Source: CAD feature listing. Evaluate the final solid. Frame: model axes, mm. A direction names the side the tool comes from. Give positions to 0.01 mm unless a question says otherwise; leave off trailing zeros. Loops run counter-clockwise (first coordinate to the right, second up) from the corner with the lowest first, then second, coordinate; pieces in that order, holes last.
from build123d import *

# Parameters (mm, degrees)
ESQUISSE1_W             = 25
ESQUISSE1_H             = 20
ESQUISSE1_R             = 1.4
ESQUISSE1_R_2           = 0.875
BOSS_EXTRU_1_DEPTH      = 3
BOSS_EXTRU_2_DEPTH      = 6
ENL_V_MAT_EXTRU_1_DEPTH = 6
ESQUISSE4_R             = 2
ENL_V_MAT_EXTRU_2_DEPTH = 1
CONG_1_R                = 0.5
ESQUISSE5_R             = 1.4
ENL_V_MAT_EXTRU_3_DEPTH = 6


with BuildPart() as part:
    # Esquisse1 → Boss.-Extru.1 (new body)
    with BuildSketch(Plane.XY):
        with Locations((12.5, 10)):
            Rectangle(ESQUISSE1_W, ESQUISSE1_H)
        with Locations((22.5, 17.5)):
            Circle(ESQUISSE1_R, mode=Mode.SUBTRACT)
        with Locations((14.491447915, 8)):
            Circle(ESQUISSE1_R_2, mode=Mode.SUBTRACT)
        with Locations((7.991447915, 8)):
            Circle(ESQUISSE1_R_2, mode=Mode.SUBTRACT)
    extrude(amount=BOSS_EXTRU_1_DEPTH)

    # Esquisse2 → Boss.-Extru.2 (add)
    with BuildSketch(Plane.XY.offset(3)):
        with BuildLine():
            Line((0, 2), (1.8, 2))
            Line((1.8, 2), (1.8, 12.222275421))
            ThreePointArc((1.8, 12.222275421), (2.092893219, 12.929382202), (2.8, 13.222275421))
            Line((2.8, 13.222275421), (4.491447915, 13.222275421))
            Line((4.491447915, 13.222275421), (4.491447915, 2.730724668))
            Line((4.491447915, 2.730724668), (17.991447915, 2.730724668))
            Line((17.991447915, 2.730724668), (17.991447915, 12.493838982))
            Line((17.991447915, 12.493838982), (25, 12.493838982))
            Line((25, 12.493838982), (25, 0))
            Line((25, 0), (0, 0))
            Line((0, 0), (0, 2))
        make_face()
    extrude(amount=BOSS_EXTRU_2_DEPTH)

    # Esquisse3 → Enlèv. mat.-Extru.1 (cut)
    with BuildSketch(Plane(origin=(0, 2.730724668, 0), x_dir=(1, 0, 0), z_dir=(0, 1, 0))):
        with BuildLine():
            Line((9.692490841, -8.5), (9.692490841, -7))
            ThreePointArc((9.692490841, -7), (9.838937451, -6.646446609), (10.192490841, -6.5))
            Line((10.192490841, -6.5), (10.692490841, -6.5))
            ThreePointArc((10.692490841, -6.5), (11.046044232, -6.646446609), (11.192490841, -7))
            Line((11.192490841, -7), (11.192490841, -8.5))
            ThreePointArc((11.192490841, -8.5), (11.046044232, -8.853553391), (10.692490841, -9))
            Line((10.692490841, -9), (10.192490841, -9))
            ThreePointArc((10.192490841, -9), (9.838937451, -8.853553391), (9.692490841, -8.5))
        make_face()
    extrude(amount=-ENL_V_MAT_EXTRU_1_DEPTH, mode=Mode.SUBTRACT)

    # Esquisse4 → Enlèv. mat.-Extru.2 (cut)
    with BuildSketch(Plane.ZY.offset(-1.8)):
        with Locations((6, 8)):
            Circle(ESQUISSE4_R)
    extrude(amount=-ENL_V_MAT_EXTRU_2_DEPTH, mode=Mode.SUBTRACT)

    # Congé1
    cong_1_edges = [part.edges().sort_by_distance(p)[0] for p in [
        (12.5, 20, 0),
        (25, 10, 0),
        (12.5, 0, 0),
        (0, 10, 0),
        (0, 20, 1.5),
        (25, 20, 1.5),
        (25, 0, 4.5),
        (0, 0, 4.5),
    ]]
    fillet(cong_1_edges, radius=CONG_1_R)

    # Esquisse5 → Enlèv. mat.-Extru.3 (cut)
    with BuildSketch(Plane.XZ):
        with Locations(Location((21.12309895, 5.598466424, 0), (0, 0, 270))):
            Circle(ESQUISSE5_R)
    extrude(amount=-ENL_V_MAT_EXTRU_3_DEPTH, mode=Mode.SUBTRACT)


solid = part.part
1) Reachability of faces 1 (the flat face through (1.8, 6, 5)), 2 (the flat face through (21, 6, 6)), 3 (the flat face through (9.692, 1, 8)), 4 (the flat face through (12, 11, 3)) from +Z, -Z, +X, -X, +Y, -Y: full face, straight path, thin tool, end or side. Return the list, or none.
Checks:
face 1: +Z, -X, +Y
face 2: -Y
face 3: +Y, -Y
face 4: +Z, +Y
2) Cut plane D-D (z = 4.5). Return loops of the section in (x, y).
Checks:
outline: (0, 0.5) arc R0.5 ccw to (0.5, 0) - (20.26, 0) - (20.26, 6) - (21.99, 6) - (21.99, 0) - (24.5, 0) arc R0.5 ccw to (25, 0.5) - (25, 12.49) - (17.99, 12.49) - (17.99, 2.73) - (4.49, 2.73) - (4.49, 13.22) - (2.8, 13.22) arc R1 ccw to (1.8, 12.22) - (1.8, 9.32) - (2.8, 9.32) - (2.8, 6.68) - (1.8, 6.68) - (1.8, 2) - (0, 2) - close
3) Cut plane B-B (y = 13.5). Return loops of the section in (x, z).
Checks:
outline: (0, 0.5) arc R0.5 ccw to (0.5, 0) - (24.5, 0) arc R0.5 ccw to (25, 0.5) - (25, 3) - (0, 3) - close
4) Cut plane A-A (x = 14.5). Return loops of the section in (y, z).
Checks:
outline: (0, 0.5) arc R0.5 ccw to (0.5, 0) - (7.13, 0) - (7.13, 3) - (2.73, 3) - (2.73, 9) - (0, 9) - close; (8.87, 0) - (19.5, 0) arc R0.5 ccw to (20, 0.5) - (20, 3) - (8.87, 3) - close
5) Contact query for flat-ended pins moving along their axis: P1, Ø5, axis at x = 8, z = 7.5, coming from the +Y side; P2, Ø2, axis at x = 1.5, z = 5, coming from the +Y side; P3, Ø4, axis at x = 10.5, y = 11.5, coming from the +Z side; P4, Ø1.1, axis at x = 14.49, y = 8, coming from the +Z side. Output: stop coordinate, or through.
Checks:
P1: stops at y = 2.73
P2: stops at y = 13.18
P3: stops at z = 3
P4: passes through
6) Ray query, probe 1 along X at (y, z) = (7.75, 5.5); probe 2 along Y at (x, z) = (22.5, 1.95); probe 3 along X at (y, z) = (4.25, 5.75). Return the intervals inside material, ascending.
Checks:
probe 1: x = 2.8 to 4.49, 17.99 to 25
probe 2: y = 0 to 16.1, 18.9 to 20
probe 3: x = 1.8 to 4.49, 17.99 to 19.73, 22.51 to 25
7) Pull-direction query (Y, two-part tool) for faces 5 (the flat face through (21, 12.494, 6)), 6 (the flat face through (12, 10, 0)), 7 (the flat face through (2.8, 8, 6)); classes: released by +Y, released by -Y, zero draft, split by the parting line, or undercut.
Checks:
face 5: released by +Y
face 6: zero draft
face 7: undercut
8) Cut plane C-C (x = 6.25). Return loops of the section in (y, z), and give its area (3 significant figures).
Checks:
outline: (0, 0.5) arc R0.5 ccw to (0.5, 0) - (19.5, 0) arc R0.5 ccw to (20, 0.5) - (20, 3) - (2.73, 3) - (2.73, 9) - (0, 9) - close
area: 76.3 mm2
